from build123d import *

# Parameters (mm, degrees)
F2_ANGLE = 350


with BuildPart() as f2:
    # F0 (on Right) → F2 (revolve)
    with BuildSketch(Plane.YZ):
        Polygon((7.8105, 12.7), (7.8105, 0), (10.033, 0), (10.033, 2.921), (9.017, 2.921), (9.017, 11.557), (9.14731, 11.915023), (8.8265, 12.7), align=None)
    revolve(axis=Axis((0, 0, 15.063431), (0, 0, 1)), revolution_arc=F2_ANGLE)


solid = f2.part
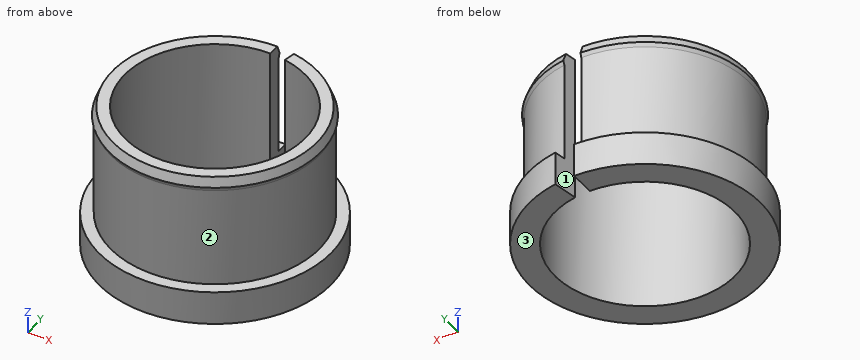
Could you check a few things on this model? Use its own coordinates, in mm. Face numbers are marked on the shaded views. Give positions to 0.01 mm unless a question says otherwise; leave off trailing zeros. Order: outer loops, then holes, each group sorted by start corner. A loop starts at its lowest first (then second) coordinate and runs counter-clockwise, first axis right, second up. Notation, with made-up numbers: (49.5, 23) -> (93.5, 23) arc R17 cw to (93.5, 56) -> close; hole circle Ø6 at (-9.5, 42.5). An arc over 180 degrees is marked (long way). Return JSON: item names as keys, results as strings.
1. Thinking about a two-plate mould opening in X: for the marked faces 1, 2 and 3, which applies, pulls with the +X half, pulls with the -X half, needs draft (parallel to the pull), parting line crosses it, or undercut?
Answer list:
{"face 1": "undercut", "face 2": "parting line crosses it", "face 3": "needs draft"}
2. I need wall thicknesses on line 1 (X direction, y = 0, z = 4); line 2 (X direction, y = -3.5, z = 9); line 3 (Y direction, x = -1.75, z = 9.5). Which ranges of each line are inside material? Lowest first, please. Write a range as from..to.
Answer list:
{"line 1": "x = -9.02..-7.81, 7.81..9.02", "line 2": "x = -8.31..-6.98, 6.98..8.31", "line 3": "y = -8.85..-7.61, 7.61..8.85"}
3. Imagine slicing it at A-A on y = 0. List the corners of the cut face in (x, z) for me, then the cut area to 3 significant figures.
Answer list:
{"outline": "(-10.03, 0) -> (-7.81, 0) -> (-7.81, 12.7) -> (-8.83, 12.7) -> (-9.15, 11.92) -> (-9.02, 11.56) -> (-9.02, 2.92) -> (-10.03, 2.92) -> close; (7.81, 0) -> (10.03, 0) -> (10.03, 2.92) -> (9.02, 2.92) -> (9.02, 11.56) -> (9.15, 11.92) -> (8.83, 12.7) -> (7.81, 12.7) -> close", "area": "36.6 mm2"}
4. For pin 1 Ø1.1 at (y, z) = (8.5, 7) entering from +X; pin 2 Ø4 at (x, z) = (4.5, 2) entering from -Y; pin 3 Ø6 at (x, z) = (0.5, 7) entering from +Y, each with a flat end and sliding along its axis, tell me the tip position at first contact or that it passes through.
Answer list:
{"pin 1": "stops at x = 4.25", "pin 2": "stops at y = -9.72", "pin 3": "stops at y = 9.02"}
5. Imagine slicing it at B-B on z = 1.5. List the corners of the cut face in (x, y) for me, then the cut area to 3 significant figures.
Answer list:
{"outline": "(0, 7.81) -> (0, 10.03) arc R10.03 ccw (long way) to (1.74, 9.88) -> (1.36, 7.69) arc R7.81 cw (long way) to start", "area": "121 mm2"}
6. Imagine slicing it at C-C on z = 7. List the corners of the cut face in (x, y) for me, then the cut area to 3 significant figures.
Answer list:
{"outline": "(0, 7.81) -> (0, 9.02) arc R9.02 ccw (long way) to (1.57, 8.88) -> (1.36, 7.69) arc R7.81 cw (long way) to start", "area": "62.0 mm2"}
